from build123d import *

# Parameters (mm, degrees)
SKETCH1_W           = 35.306
SKETCH1_H           = 35.306
BOSS_EXTRUDE1_DEPTH = 34.036
SKETCH2_R           = 10.9982
BOSS_EXTRUDE2_DEPTH = 1.99898
SKETCH3_R           = 2.9972
CUT_EXTRUDE1_DEPTH  = 1.016
CHAMFER1_SIZE       = 2.54


with BuildPart() as part:
    # Sketch1 → Boss-Extrude1 (new body)
    with BuildSketch(Plane.XY):
        Rectangle(SKETCH1_W, SKETCH1_H)
    extrude(amount=BOSS_EXTRUDE1_DEPTH)

    # Sketch2 → Boss-Extrude2 (add)
    with BuildSketch(Plane.XY.offset(34.036)):
        Circle(SKETCH2_R)
    extrude(amount=BOSS_EXTRUDE2_DEPTH)

    # Sketch3 → Cut-Extrude1 (cut)
    with BuildSketch(Plane.XY.offset(36.03498)):
        Circle(SKETCH3_R)
    extrude(amount=-CUT_EXTRUDE1_DEPTH, mode=Mode.SUBTRACT)

    # Chamfer1
    chamfer1_edges = [part.edges().sort_by_distance(p)[0] for p in [
        (-17.653, 17.653, 17.018),
        (17.653, 17.653, 17.018),
        (17.653, -17.653, 17.018),
        (-17.653, -17.653, 17.018),
    ]]
    chamfer(chamfer1_edges, length=CHAMFER1_SIZE)


solid = part.part
Geometry: final body of the model. Coordinates: model frame, mm. A direction names the side the tool comes from. Round coordinates to 2 decimals unless told otherwise and drop trailing zeros. Loops run counter-clockwise (first coordinate to the right, second up) from the corner with the lowest first, then second, coordinate; pieces in that order, holes last.
Q1. Section D-D on y = 8.5. Return loops of the section in (x, z), plus the area to 3 significant figures.
Q2. Section A-A on x = 0. Return loops of the section in (y, z).
Q3. Access query for faces 4 (the cylindrical face through (-8.73, -6.69, 35.02)), 5 (the flat face through (-16.365, -16.401, 16.78)). Directions: +Z, -Z, +X, -X, +Y, -Y. A direction counts if a zero-diameter tool reaches every point of the face in a straight line with its end or side. Return the directions, or none.
Q4. Material intervals for L1, parallel to Y at x = 0, z = 35.3; L2, parallel to Z at x = -6.5, y = 11; L3, parallel to Z at x = -2.5, y = -0.5, sorted ascending.
Q5. Section C-C on x = 14.5. Return loops of the section in (y, z), plus the area to 3 significant figures.
Q6. Pin query (flat end, axial travel): P1, Ø9.5, axis at x = 0, y = 0, coming from the +Z side (3 decimals); P2, Ø3, axis at x = 1, y = 0.5, coming from the +Z side; P3, Ø6, axis at x = 13.5, y = -10.5, coming from the +Z side. Return the tip coordinate at first contact, or that it passes through.
Q7. Pull-direction query (Y, two-part tool) for faces 1 (the flat face through (0, 0, 35.019)), 2 (the flat face through (0, 17.653, 17)), 3 (the flat face through (16.401, -16.365, 16.78)); classes: released by +Y, released by -Y, zero draft, split by the parting line, or undercut.
Evaluation:
1. outline: (-17.65, 0) - (17.65, 0) - (17.65, 34.04) - (6.98, 34.04) - (6.98, 36.03) - (-6.98, 36.03) - (-6.98, 34.04) - (-17.65, 34.04) - close
1. area: 1,230 mm2
2. outline: (-17.65, 0) - (17.65, 0) - (17.65, 34.04) - (11, 34.04) - (11, 36.03) - (3, 36.03) - (3, 35.02) - (-3, 35.02) - (-3, 36.03) - (-11, 36.03) - (-11, 34.04) - (-17.65, 34.04) - close
3. face 4: +Z
3. face 5: +Z, -Z, -X, -Y
4. L1: y = -11 to -3, 3 to 11
4. L2: z = 0 to 34.04
4. L3: z = 0 to 35.02
5. outline: (-17.65, 0) - (17.65, 0) - (17.65, 34.04) - (-17.65, 34.04) - close
5. area: 1,200 mm2
6. P1: stops at z = 36.035
6. P2: stops at z = 35.02
6. P3: stops at z = 34.04
7. face 1: undercut
7. face 2: released by +Y
7. face 3: released by -Y
